Answer from the drawing. Dimensions are ordinates in mm from the lowest x, y and z of the part. Coordinates: 2 decimals unless noted, no trailing zeros. Write each loop counter-clockwise with the first axis right and the second up, starting at its lowest first coordinate (ties: lowest second). Pieces come first, ordered by that corner, then holes. Notation, with made-up numbers: (-20, 30) - (30, 30) arc R17 cw to (30, 34) - close; hole circle Ø2 at (69, 41). An arc over 180 degrees is marked (long way). Use one line per item in the form item = value. Start each with the question number.
Item 1: A cutting plane is placed at D-D (z = 2.5). Write down the section's boundary in (x, y).
Item 2: Consider probe 1 along X at (y, z) = (1.5, 16.5). Determine where the line is inside the solid, lowest interval first.
Item 3: Given pin 1 (0.5 mm diameter, centred on y = 6, z = 17.5, fed in from -X); pin 2 (1.1 mm diameter, centred on x = 0.5, y = 6, fed in from -Z); pin 3 (0.8 mm diameter, centred on y = 5, z = 0.5, fed in from -X); pin 4 (0.5 mm diameter, centred on y = 11.5, z = 0.5, fed in from -X), each flat-ended and moving along its own axis, determine where each tip first touches the part or whether it passes through.
Item 4: A cutting plane is placed at B-B (x = 11.5). Write down the section's boundary in (y, z).
Item 5: A cutting plane is placed at A-A (z = 10.25). Write down the section's boundary in (x, y).
Item 6: A cutting plane is placed at C-C (y = 9.25). Write down the section's boundary in (x, z).
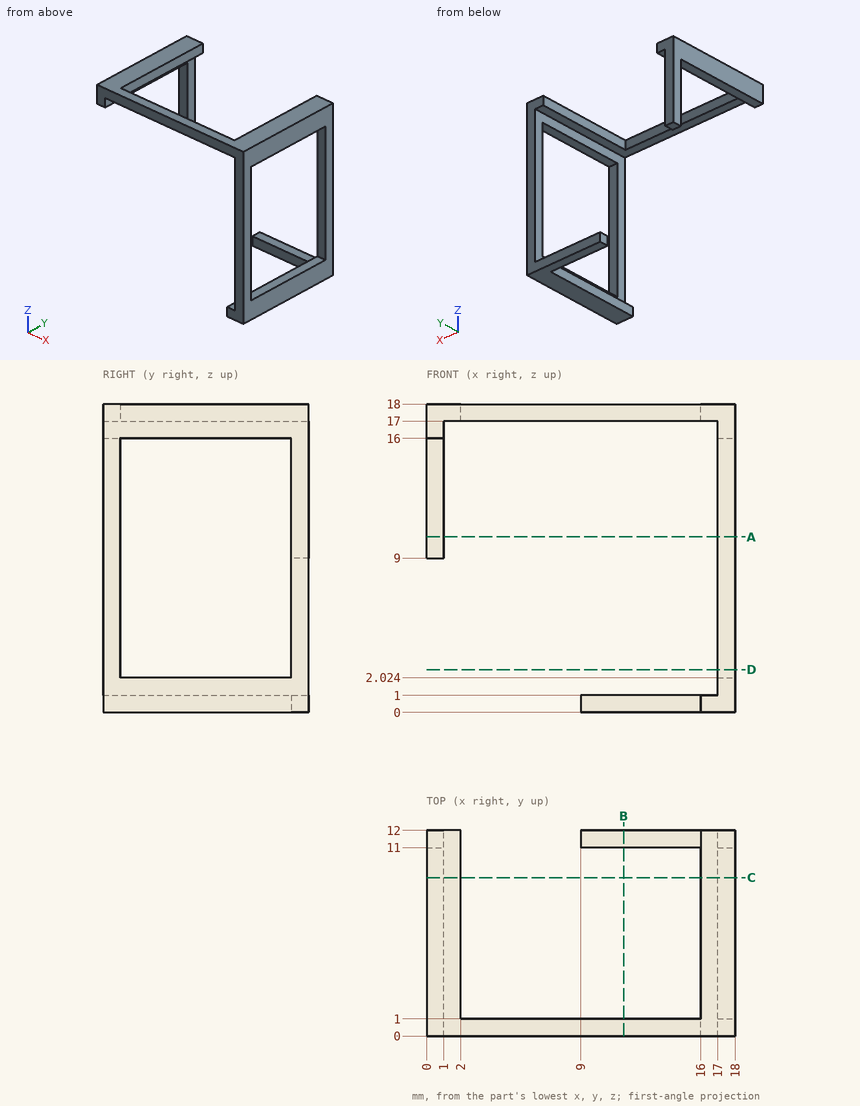
Answer:
q1.outline = (17, 0) - (18, 0) - (18, 1) - (17, 1) - close; (17, 11) - (18, 11) - (18, 12) - (17, 12) - close
q2.probe_1 = 0 to 1, 17 to 18
q3.pin_1 = 0
q3.pin_2 = 16
q3.pin_3 = 16
q3.pin_4 = 9
q4.outline = (0, 17) - (1, 17) - (1, 18) - (0, 18) - close; (11, 0) - (12, 0) - (12, 1) - (11, 1) - close
q5.outline = (0, 11) - (1, 11) - (1, 12) - (0, 12) - close; (17, 0) - (18, 0) - (18, 1) - (17, 1) - close; (17, 11) - (18, 11) - (18, 12) - (17, 12) - close
q6.outline = (0, 16) - (1, 16) - (1, 17) - (2, 17) - (2, 18) - (0, 18) - close; (16, 0) - (18, 0) - (18, 2.02) - (17, 2.02) - (17, 1) - (16, 1) - close; (16, 17) - (17, 17) - (17, 16) - (18, 16) - (18, 18) - (16, 18) - close
